Can you work these out from the drawing? Everything is in mm from the part's minimum corner. Give positions to 0.01 mm unless a question says otherwise; leave off trailing zeros. Order: outer loops, then holes, each group sorted by start corner. A loop starts at its lowest first (then second) coordinate and runs counter-clockwise, first axis right, second up. Notation, with made-up numbers: (71, -12) -> (96, -12) arc R26 cw to (96, 15) -> close; hole circle Ø8 at (28, 30.5). An arc over 180 degrees is marked (long way). Answer as CSV lines item,"result". Start each with the question number.
(1) I want a section at C-C (z = 3.81). Please give me the cut outline in (x, y), plus the area to 3 significant figures.
(2) I want a section at B-B (y = 3.81). Please give me the cut outline in (x, z), plus the area to 3 significant figures.
(3) Will these pins go through, and if not, where does the flat tip stop? pin 1 Ø3 at (y, z) = (3.81, 3.81) entering from -X; pin 2 Ø2.5 at (y, z) = (53.34, 3.81) entering from +X.
(4) I want a section at A-A (x = 0.9). Please give me the cut outline in (y, z).
(5) I need wall thicknesses on L1, parallel to Z at x = 0.6, y = 3.81; L2, parallel to Y at x = 0.1, z = 15.75. Which ranges of each line are inside material? Lowest first, please.
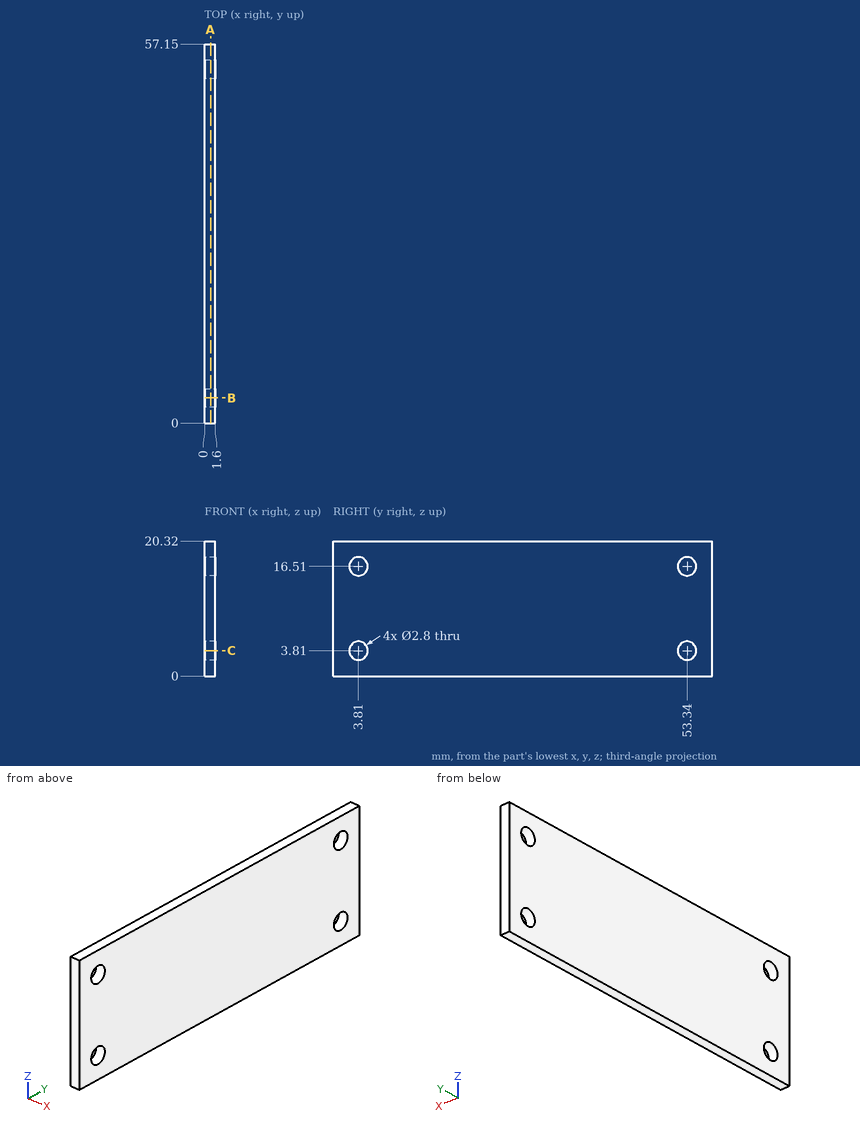
Final values:
1,outline,"(0, 0) -> (1.6, 0) -> (1.6, 2.41) -> (0, 2.41) -> close; (0, 5.21) -> (1.6, 5.21) -> (1.6, 51.94) -> (0, 51.94) -> close; (0, 54.74) -> (1.6, 54.74) -> (1.6, 57.15) -> (0, 57.15) -> close"
1,area,"82.5 mm²"
2,outline,"(0, 0) -> (1.6, 0) -> (1.6, 2.41) -> (0, 2.41) -> close; (0, 5.21) -> (1.6, 5.21) -> (1.6, 15.11) -> (0, 15.11) -> close; (0, 17.91) -> (1.6, 17.91) -> (1.6, 20.32) -> (0, 20.32) -> close"
2,area,"23.6 mm²"
3,pin 1,"x = 0"
3,pin 2,"through"
4,outline,"(0, 0) -> (57.15, 0) -> (57.15, 20.32) -> (0, 20.32) -> close; hole circle Ø2.8 at (3.81, 3.81); hole circle Ø2.8 at (3.81, 16.51); hole circle Ø2.8 at (53.34, 3.81); hole circle Ø2.8 at (53.34, 16.51)"
5,L1,"0 to 2.41, 5.21 to 15.11, 17.91 to 20.32"
5,L2,"0 to 2.63, 4.99 to 52.16, 54.52 to 57.15"
